from build123d import *

# Parameters (mm, degrees)
F0_W     = 4
F0_H     = 17.5
F0_R     = 7.5
F0_H_2   = 17
F1_DEPTH = 4


with BuildPart() as f1:
    # F0 (on Top) → F1 (new body)
    with BuildSketch(Plane.XY):
        Polygon((9, 0), (0, 0), (0, -26.5), (26.75, -26.5), (31.95, -26.5), (31.95, -22.5), (76.45, -22.5), (76.45, -26.5), (79.75, -26.5), (99.5, -26.5), (99.5, -6.7), (97.5, -6.7), (97.5, -10.7), (93.5, -10.7), (93.5, 1.444), (57.45, 1.444), (50.5, 9), (40.5, 9), (40.5, 0), (13, 0), (13, -9), (9, -9), align=None)
        with Locations((4.4, -13.75)):
            Rectangle(F0_W, F0_H, mode=Mode.SUBTRACT)
        with Locations((21.5, -15)):
            Circle(F0_R, mode=Mode.SUBTRACT)
        with Locations((81.5, -15)):
            Circle(F0_R, mode=Mode.SUBTRACT)
        with Locations((61, -10)):
            Rectangle(F0_W, F0_H_2, mode=Mode.SUBTRACT)
        Polygon((31.95, -26.5), (26.75, -26.5), (26.75, -29.5), (79.75, -29.5), (79.75, -26.5), (76.45, -26.5), align=None)
    extrude(amount=F1_DEPTH)


solid = f1.part
Verification items for the finished model (mm, model axes). A direction names the side the tool comes from. Give positions to 0.01 mm unless a question says otherwise; leave off trailing zeros. Write each loop counter-clockwise with the first axis right and the second up, starting at its lowest first coordinate (ties: lowest second). Pieces come first, ordered by that corner, then holes. Notation, with made-up numbers: (-38.75, 36.25) - (15.25, 36.25) arc R17 ccw to (15.25, 54.25) - close; hole circle Ø9 at (7.5, -22). An arc over 180 degrees is marked (long way). Answer as CSV lines item,"result". Start each with the question number.
1. Sectioned sample at D-D (z = 2.25). Count the separate pieces of the cut face and the enclosed holes in it, then the cut area to 3 significant figures.
2. Sectioned sample at B-B (y = -15). Record the boundary of the cut face in (x, z), then the cut area to 3 significant figures.
3. Draft check along X on faces 1 (the face through (79.75, -28, 2)), 2 (the face through (97.5, -9, 2)), 3 (the face through (53, -29.5, 2)). Enter one of: pulls with the +X half, pulls with the -X half, needs draft (parallel to the pull), parting line crosses it, or undercut.
4. Sectioned sample at C-C (y = -2.5). Record the boundary of the cut face in (x, z), then the cut area to 3 significant figures.
5. Set-up check for faces 4 (the face through (96, -10.7, 2)), 5 (the face through (13, -26.5, 2)), 6 (the face through (4, -5, 2)), 7 (the face through (99, -6.7, 2)), 8 (the face through (89, -26.5, 2)): record each of +Z, -Z, +X, -X, +Y, -Y from which the full face is reachable in a straight line by a thin tool's end or side.
6. Depth check by flat-ended pin: pin 1 (13.5 mm diameter, centred on x = 81.5, y = -15, fed in from +Z); pin 2 (1.2 mm diameter, centred on x = 53.5, z = 2.5, fed in from +Y); pin 3 (1.6 mm diameter, centred on x = 99, z = 3, fed in from +Y). Enter the tip coordinate at first touch or a pass-through.
7. Sectioned sample at A-A (x = 21.5). Record the boundary of the cut face in (y, z).
8. Thickness scan on line 1 (X direction, y = -3.5, z = 3.45); line 2 (X direction, y = -15.5, z = 1.35); line 3 (X direction, y = -19, z = 0.4). Record the ranges inside material, lowest first.
Derived:
1,separate pieces,"1"
1,enclosed holes,"5"
1,area,"2,210 mm²"
2,outline,"(0, 0) - (2.4, 0) - (2.4, 4) - (0, 4) - close; (6.4, 0) - (14, 0) - (14, 4) - (6.4, 4) - close; (29, 0) - (59, 0) - (59, 4) - (29, 4) - close; (63, 0) - (74, 0) - (74, 4) - (63, 4) - close; (89, 0) - (99.5, 0) - (99.5, 4) - (89, 4) - close"
2,area,"246 mm²"
3,face 1,"pulls with the +X half"
3,face 2,"undercut"
3,face 3,"needs draft"
4,outline,"(0, 0) - (9, 0) - (9, 4) - (0, 4) - close; (13, 0) - (59, 0) - (59, 4) - (13, 4) - close; (63, 0) - (93.5, 0) - (93.5, 4) - (63, 4) - close"
4,area,"342 mm²"
5,face 4,"+Z, -Z, +Y"
5,face 5,"+Z, -Z, -X, -Y"
5,face 6,"+Z, -Z"
5,face 7,"+Z, -Z, +X, +Y"
5,face 8,"+Z, -Z, +X, -Y"
6,pin 1,"through"
6,pin 2,"y = 6.39"
6,pin 3,"y = -6.7"
7,outline,"(-26.5, 0) - (-22.5, 0) - (-22.5, 4) - (-26.5, 4) - close; (-7.5, 0) - (0, 0) - (0, 4) - (-7.5, 4) - close"
8,line 1,"0 to 9, 13 to 59, 63 to 93.5"
8,line 2,"0 to 2.4, 6.4 to 14.02, 28.98 to 59, 63 to 74.02, 88.98 to 99.5"
8,line 3,"0 to 2.4, 6.4 to 15.16, 27.84 to 75.16, 87.84 to 99.5"
